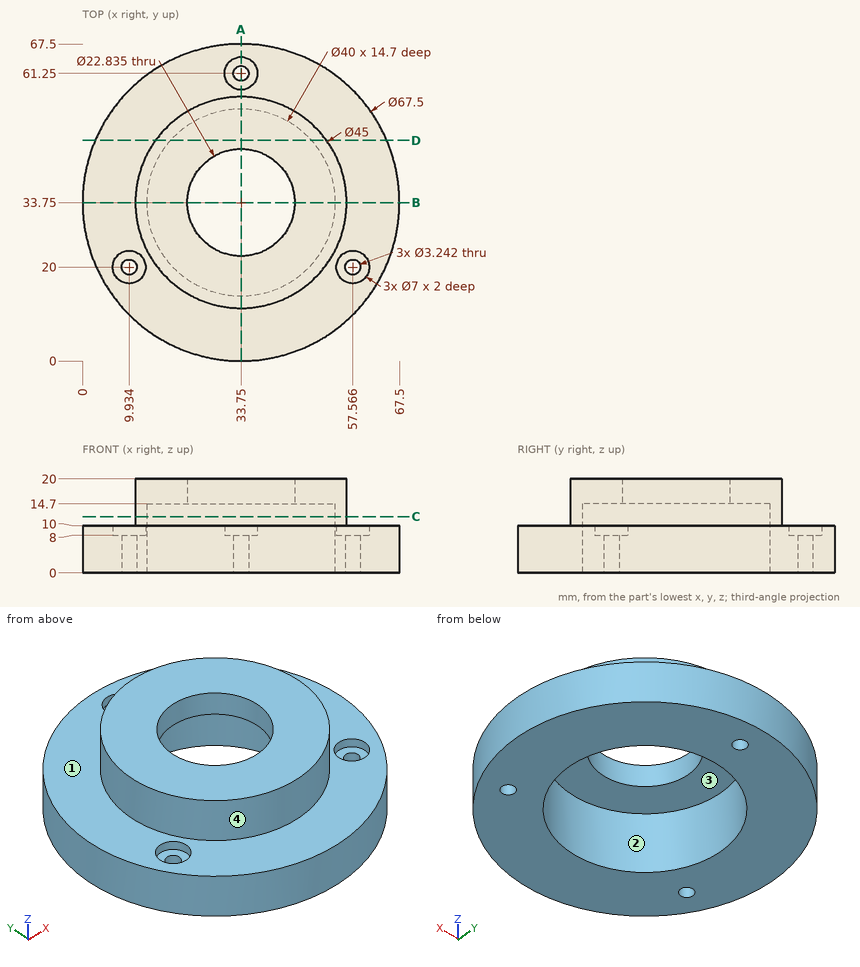
Check sheet for the drawn part. Datum: minimum x, y, z corner. Units: mm. Coordinates: 2 decimals unless noted, no trailing zeros. Loops run counter-clockwise (first coordinate to the right, second up) from the corner with the lowest first, then second, coordinate; pieces in that order, holes last. Notation, with made-up numbers: (40, 78) - (58, 78) arc R23 cw to (58, 116) - close; hole circle Ø3 at (-18.75, 7.5). An arc over 180 degrees is marked (long way). Put each result on its own line as item: value.
Item 1: Section check C-C (z = 12). Enter the section's corners in (x, y).
Conclusion:
outline: circle Ø45 at (33.75, 33.75); hole circle Ø40 at (33.75, 33.75)
Item 2: Draft check along X on the marked faces 1, 2, 3 and 4. Enter one of: pulls with the +X half, pulls with the -X half, needs draft (parallel to the pull), parting line crosses it, or undercut.
Conclusion:
face 1: needs draft
face 2: undercut
face 3: undercut
face 4: parting line crosses it
Item 3: Section check D-D (y = 47). Enter the section's corners in (x, z) (1 decimal).
Conclusion:
outline: (2.7, 0) - (18.8, 0) - (18.8, 14.7) - (48.7, 14.7) - (48.7, 0) - (64.8, 0) - (64.8, 10) - (51.9, 10) - (51.9, 20) - (15.6, 20) - (15.6, 10) - (2.7, 10) - close
Item 4: Gauge pin test, flat ends, axial feed: pin 1 Ø2 at (x, z) = (10, 9) entering from +Y; pin 2 Ø1.9 at (x, y) = (9.93, 20) entering from +Z; pin 3 Ø2 at (y, z) = (13.5, 4) entering from +X; pin 4 Ø3.5 at (x, y) = (57, 20) entering from +Z. Record the tip position at first contact, or that the pin passes through.
Conclusion:
pin 1: stops at y = 58.68
pin 2: passes through
pin 3: stops at x = 61.47
pin 4: stops at z = 8
Item 5: Section check A-A (x = 33.75). Enter the section's corners in (y, z).
Conclusion:
outline: (0, 0) - (13.75, 0) - (13.75, 14.7) - (22.33, 14.7) - (22.33, 20) - (11.25, 20) - (11.25, 10) - (0, 10) - close; (45.17, 14.7) - (53.75, 14.7) - (53.75, 0) - (59.63, 0) - (59.63, 8) - (57.75, 8) - (57.75, 10) - (56.25, 10) - (56.25, 20) - (45.17, 20) - close; (62.87, 0) - (67.5, 0) - (67.5, 10) - (64.75, 10) - (64.75, 8) - (62.87, 8) - close
Item 6: Section check B-B (y = 33.75). Enter the section's corners in (x, z), then the cut area to 3 significant figures.
Conclusion:
outline: (0, 0) - (13.75, 0) - (13.75, 14.7) - (22.33, 14.7) - (22.33, 20) - (11.25, 20) - (11.25, 10) - (0, 10) - close; (45.17, 14.7) - (53.75, 14.7) - (53.75, 0) - (67.5, 0) - (67.5, 10) - (56.25, 10) - (56.25, 20) - (45.17, 20) - close
area: 416 mm2
Item 7: Scan lines: line 1 along Y through (x, z) = (34.5, 9); line 2 along Z through (x, y) = (42, 59); line 3 along Z through (x, y) = (19, 32). Record each from-to range of solid material in increasing order.
Conclusion:
line 1: y = 0.01 to 13.76, 53.74 to 57.83, 64.67 to 67.49
line 2: z = 0 to 10
line 3: z = 14.7 to 20
